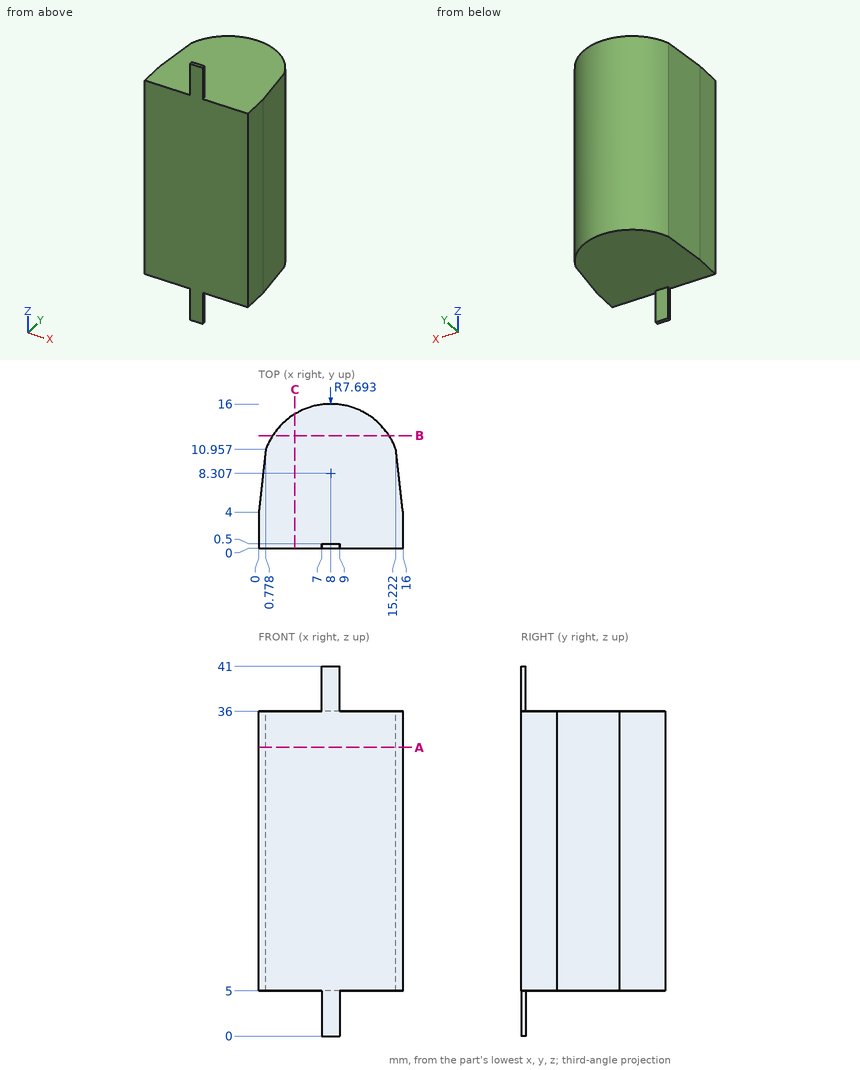
Part print with two shaded views. Sizes in mm from the minimum x, y, z corner. Coordinates: 2 decimals unless noted, no trailing zeros. Write each loop counter-clockwise with the first axis right and the second up, starting at its lowest first coordinate (ties: lowest second). Pieces come first, ordered by that corner, then holes.
(1) Cut at A-A on z = 32. List the corners of the cut face in (x, y), and give its area (3 significant figures).
(2) Cut at B-B on y = 12.5. List the corners of the cut face in (x, z).
(3) Pin check, flat tips, straight feed: pin 1 Ø5 at (x, y) = (4, 7.5) entering from +Z; pin 2 Ø4 at (x, y) = (12, 6) entering from -Z; pin 3 Ø0.6 at (y, z) = (0.5, 39) entering from +X. Stop position of each tip, or through.
(4) Cut at C-C on x = 4. List the corners of the cut face in (y, z), and give its area (3 significant figures).
(5) Drill centre lines: line 1 (Z direction, x = 5.75, y = 11.5); line 2 (Y direction, x = 7.75, z = 26); line 3 (X direction, y = 13.5, z = 7.5) (1 decimal). Where is each one in solid material? Low to high.
Working result:
1. outline: (0, 0) - (16, 0) - (16, 4) - (15.22, 10.96) arc R7.69 ccw to (0.78, 10.96) - (0, 4) - close
1. area: 223 mm2
2. outline: (1.55, 5) - (14.45, 5) - (14.45, 36) - (1.55, 36) - close
3. pin 1: stops at z = 36
3. pin 2: stops at z = 5
3. pin 3: stops at x = 9
4. outline: (0, 5) - (14.88, 5) - (14.88, 36) - (0, 36) - close
4. area: 461 mm2
5. line 1: z = 5 to 36
5. line 2: y = 0 to 16
5. line 3: x = 2.3 to 13.7
